The drawing under review shows one solid part. Ordinate dimensions are in mm from its lowest x, y, z. Coordinates: 2 decimals unless noted, no trailing zeros. Loops run counter-clockwise (first coordinate to the right, second up) from the corner with the lowest first, then second, coordinate; pieces in that order, holes last. Notation, with made-up numbers: M 72.5,-18.75 L 96.5,-18.75 A19 cw 96.5,-12.75 Z; hole C -17.75,62.25 d9. An arc over 180 degrees is marked long. Answer as a JSON object with one key per item and string values. Group by question number.
1. Consider section A-A (z = 2.5). Count the separate pieces of the cut face and the enclosed holes in it, then the cut area to 3 significant figures.
2. To check wall thickness, follow probe 1 along X at (y, z) = (2.75, 2.75) (1 decimal); probe 2 along X at (y, z) = (7.75, 2.5) (1 decimal); probe 3 along X at (y, z) = (5.5, 3.5). State the ranges of each line that lie inside material, in increasing order.
3. Draft analysis for pull direction X (two halves, no side actions). For the marked faces 1, 2, 3 and 4, state which applies: +X half, -X half, draft (parallel to the pull), parting line (faces both ways), or undercut.
4. Insertion check: pin 1 (1 mm diameter, centred on x = 39.5, z = 1.5, fed in from -Y); pin 2 (5 mm diameter, centred on x = 44.45, y = 6.35, fed in from -Z); pin 3 (1 mm diameter, centred on x = 13.5, y = 5, fed in from -Z) (1 decimal). Each pin has a flat end and moves straight along its axis. Give the tip position at first contact, or say it passes through.
5. Consider section B-B (x = 44.45). State the section outline as (y, z) points (1 decimal).
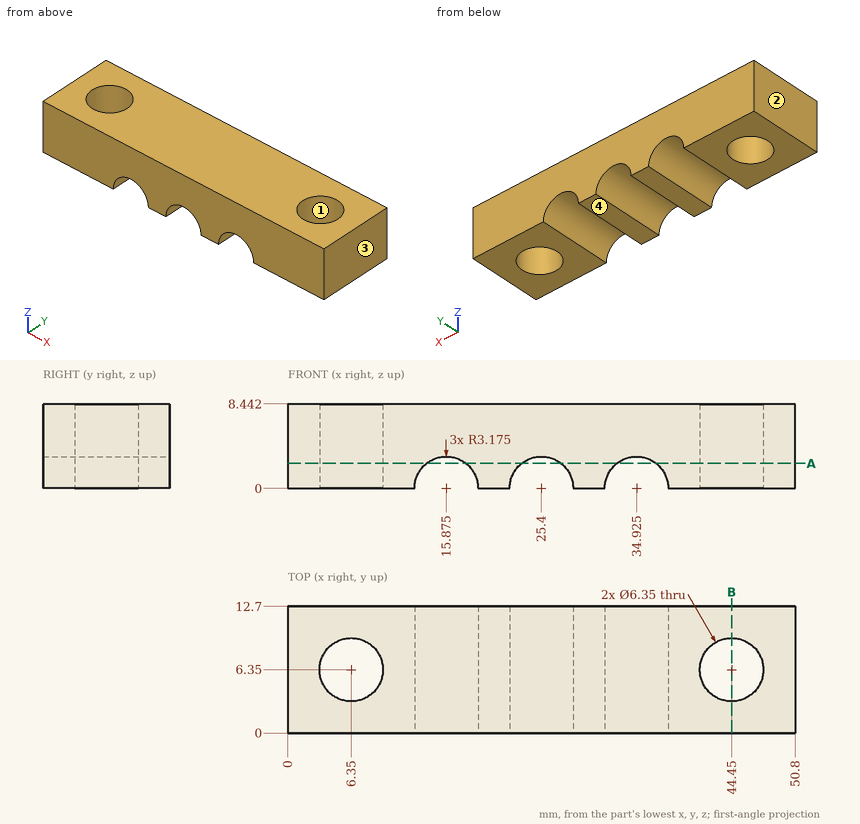
Findings below:
{
 "1": {"separate pieces": "4", "enclosed holes": "2", "area": "433 mm^2"},
 "2": {"probe 1": "x = 0 to 14.3, 17.5 to 23.8, 27 to 33.3, 36.5 to 50.8", "probe 2": "x = 0 to 3.5, 9.2 to 13.9, 17.8 to 23.4, 27.4 to 33, 36.9 to 41.6, 47.3 to 50.8", "probe 3": "x = 0 to 3.29, 9.41 to 41.39, 47.51 to 50.8"},
 "3": {"face 1": "undercut", "face 2": "-X half", "face 3": "+X half", "face 4": "draft"},
 "4": {"pin 1": "stops at y = 0", "pin 2": "passes through", "pin 3": "stops at z = 1.3"},
 "5": {"outline": "M 0,0 L 3.2,0 L 3.2,8.4 L 0,8.4 Z; M 9.5,0 L 12.7,0 L 12.7,8.4 L 9.5,8.4 Z"}
}
